Part model, mm, in its own coordinate system. Face numbers are marked on the shaded views. A direction names the side the tool comes from. Round coordinates to 2 decimals unless told otherwise and drop trailing zeros. Loops run counter-clockwise (first coordinate to the right, second up) from the corner with the lowest first, then second, coordinate; pieces in that order, holes last. Notation, with made-up numbers: M 76,46.25 L 127,46.25 A9 cw 127,51.25 Z; hole C 50.5,33.5 d10. An arc over 180 degrees is marked long. Answer as CSV lines item,"result". Start each with the question number.
Item 1: Band-saw the part on D-D (x = 39.5). Give the cut face in (y, z) (3 decimals), and give its area (3 significant figures).
Item 2: Which spindle directions (+Z, -Z, +X, -X, +Y, -Y) get a long thin tool onto all of the face, cutting with end or side? Do the marked faces 4, 5 and 6. Say none if no direction does.
Item 3: Band-saw the part on B-B (z = 6.5). Give the cut face in (x, y) (3 decimals).
Item 4: Mould opens along X. For the marked faces 1, 2 and 3 say: pulls with the +X half, pulls with the -X half, needs draft (parallel to the pull), parting line crosses it, or undercut.
Item 5: Band-saw the part on A-A (x = 12). Give the cut face in (y, z) (3 decimals).
Item 6: Band-saw the part on C-C (z = 12). Give the cut face in (x, y) (3 decimals), and give its area (3 significant figures).
Item 7: Drop flat-ended pins along their axis: pin 1 Ø3 at (x, y) = (13, -7) entering from -Z; pin 2 Ø3 at (y, z) = (-6.5, 7) entering from +X; pin 3 Ø5 at (x, y) = (12, -6) entering from +Z. Give the stop position or say it passes through.
Item 8: Wall check: line 1 (X direction, y = -6, z = 8.5); line 2 (Y direction, x = 31.5, z = 10.75). Give the ranges that are in metal, low to high.
```python
from build123d import *

# Parameters (mm, degrees)
F0_W     = 53.34
F0_H     = 68.58
F1_DEPTH = 15.875
F2_W     = 12.443692
F2_H     = 11.007975
F2_R     = 4.449161
F3_DEPTH = 9.525


with BuildPart() as f1:
    # F0 (on Top) → F1 (new body)
    with BuildSketch(Plane.XY):
        with Locations((26.67, 34.29)):
            Rectangle(F0_W, F0_H)
    extrude(amount=F1_DEPTH)

    # F2 (on face) → F3 (join)
    with BuildSketch(Plane.XZ):
        with Locations((13.379577, 8.078674)):
            Rectangle(F2_W, F2_H)
        with Locations((42.665571, 8.831811)):
            Circle(F2_R)
    extrude(amount=F3_DEPTH)


solid = f1.part
```
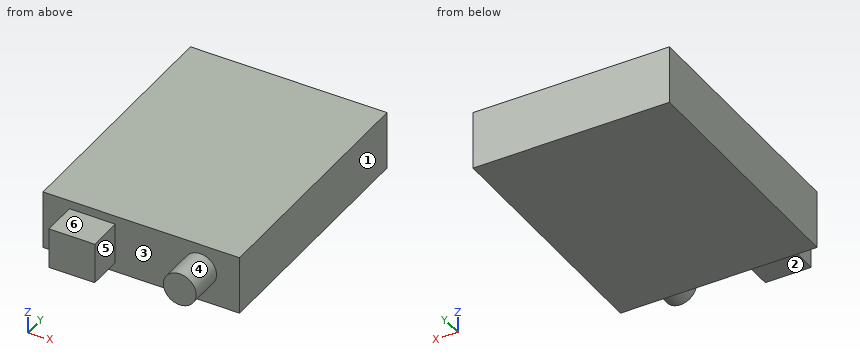
Answer block:
1,outline,"M -9.525,5.705 L 0,5.705 L 0,0 L 68.58,0 L 68.58,15.875 L 0,15.875 L 0,11.958 L -9.525,11.958 Z"
1,area,"1,150 mm^2"
2,face 4,"-Y"
2,face 5,"+Z, -Z, -Y"
2,face 6,"+Z, +X, -X, -Y"
3,outline,"M 0,0 L 7.158,0 L 7.158,-9.525 L 19.601,-9.525 L 19.601,0 L 38.876,0 L 38.876,-9.525 L 46.455,-9.525 L 46.455,0 L 53.34,0 L 53.34,68.58 L 0,68.58 Z"
4,face 1,"pulls with the +X half"
4,face 2,"needs draft"
4,face 3,"undercut"
5,outline,"M -9.525,2.575 L 0,2.575 L 0,0 L 68.58,0 L 68.58,15.875 L 0,15.875 L 0,13.583 L -9.525,13.583 Z"
6,outline,"M 0,0 L 7.158,0 L 7.158,-9.525 L 19.601,-9.525 L 19.601,0 L 39.542,0 L 39.542,-9.525 L 45.789,-9.525 L 45.789,0 L 53.34,0 L 53.34,68.58 L 0,68.58 Z"
6,area,"3,840 mm^2"
7,pin 1,"stops at z = 2.57"
7,pin 2,"stops at x = 47.1"
7,pin 3,"stops at z = 13.58"
8,line 1,"x = 7.16 to 19.6, 38.23 to 47.1"
8,line 2,"y = 0 to 68.58"
